The listing builds one solid part. Answer for the finished solid, in the listing's coordinates (mm). A direction names the side the tool comes from. Give positions to 0.01 mm unless a question says otherwise; leave off trailing zeros. Loops run counter-clockwise (first coordinate to the right, second up) from the corner with the lowest first, then second, coordinate; pieces in that order, holes last.
Item 1: Section B-B, the plane z = 19.05 is taken. Give the vertices of the cut face in (x, y), and give its area (3 significant figures).
Item 2: A tool of negligible diameter and unlimited length cuts with its end or side. For faces 1 (the face through (10.878, 1, 9)), 2 (the face through (-6.6, 2, 0)), 3 (the face through (17, 2.2, 21)), from which of +Z, -Z, +X, -X, +Y, -Y can it reach the whole face along a straight path? Write none if from no direction.
Item 3: Section C-C, the plane x = 0 is taken. Give the vertices of the cut face in (y, z).
Item 4: Consider line 1 along Z through (x, y) = (19.05, 1.3); line 2 along X through (y, z) = (3.25, -17.5). Determine where each line is inside the solid, lowest interval first.
Item 5: Section D-D, the plane z = 8.5 is taken. Give the vertices of the cut face in (x, y).
Item 6: The mould has two halves that part along Z. Classify faces 4 (the face through (-24.19, 2.54, -24.15)), 5 (the face through (10.878, 1, -9)): pulls with the +Z half, pulls with the -Z half, needs draft (parallel to the pull), parting line crosses it, or undercut.
Item 7: Each of these flat-tipped pins is pushed along its axis until it touches: pin 1 Ø6 at (x, z) = (19.05, 19.05) entering from +Y; pin 2 Ø1.6 at (x, z) = (8, -7) entering from -Y. Where does it stop, or does it pass through?
Item 8: Section A-A, the plane x = 19.05 is taken. Give the vertices of the cut face in (y, z), and give its area (3 significant figures).
from build123d import *

# Parameters (mm, degrees)
SKETCH1_W           = 50.1
SKETCH1_H           = 50.1
SKETCH1_R           = 1.7
SKETCH1_R_2         = 2.5527
SKETCH1_W_2         = 13.2
SKETCH1_H_2         = 6.8
BOSS_EXTRUDE1_DEPTH = 5
FILLET1_R           = 3
CUT_EXTRUDE1_DEPTH  = 2.6
SKETCH5_R           = 4.5675
CUT_EXTRUDE4_DEPTH  = 2.8
FILLET2_R           = 0.5


with BuildPart() as part:
    # Sketch1 → Boss-Extrude1 (new body)
    with BuildSketch(Plane(origin=(0, 0, 0), x_dir=(1, 0, 0), z_dir=(0, 1, 0))):
        Rectangle(SKETCH1_W, SKETCH1_H)
        with Locations(Location((8.128, 8.5344, 0), (0, 0, 270))):
            Circle(SKETCH1_R, mode=Mode.SUBTRACT)
        with Locations(Location((-8.128, 8.5344, 0), (0, 0, 270))):
            Circle(SKETCH1_R, mode=Mode.SUBTRACT)
        with Locations(Location((19.05, 19.05, 0), (0, 0, 270))):
            Circle(SKETCH1_R_2, mode=Mode.SUBTRACT)
        with Locations(Location((-19.05, 19.05, 0), (0, 0, 270))):
            Circle(SKETCH1_R_2, mode=Mode.SUBTRACT)
        with Locations(Location((19.05, -19.05, 0), (0, 0, 270))):
            Circle(SKETCH1_R_2, mode=Mode.SUBTRACT)
        with Locations(Location((-19.05, -19.05, 0), (0, 0, 270))):
            Circle(SKETCH1_R_2, mode=Mode.SUBTRACT)
        with Locations(Location((8.128, -8.5344, 0), (0, 0, 270))):
            Circle(SKETCH1_R, mode=Mode.SUBTRACT)
        with Locations(Location((-8.128, -8.5344, 0), (0, 0, 270))):
            Circle(SKETCH1_R, mode=Mode.SUBTRACT)
        Rectangle(SKETCH1_W_2, SKETCH1_H_2, mode=Mode.SUBTRACT)
    extrude(amount=BOSS_EXTRUDE1_DEPTH)

    # Fillet1
    fillet1_edges = [part.edges().sort_by_distance(p)[0] for p in [
        (-25.05, 2.5, 25.05),
        (-25.05, 2.5, -25.05),
        (25.05, 2.5, -25.05),
        (25.05, 2.5, 25.05),
    ]]
    fillet(fillet1_edges, radius=FILLET1_R)

    # Sketch2 → Cut-Extrude1 (cut)
    with BuildSketch(Plane.XZ):
        Polygon((-8.128, 11.709826481), (-10.878, 10.12211324), (-10.878, 6.94668676), (-8.128, 5.358973519), (-5.378, 6.94668676), (-5.378, 10.12211324), align=None)
        Polygon((8.128, 11.709826481), (5.378, 10.12211324), (5.378, 6.94668676), (8.128, 5.358973519), (10.878, 6.94668676), (10.878, 10.12211324), align=None)
        Polygon((-8.128, -5.358973519), (-10.878, -6.94668676), (-10.878, -10.12211324), (-8.128, -11.709826481), (-5.378, -10.12211324), (-5.378, -6.94668676), align=None)
        Polygon((8.128, -5.358973519), (5.378, -6.94668676), (5.378, -10.12211324), (8.128, -11.709826481), (10.878, -10.12211324), (10.878, -6.94668676), align=None)
    extrude(amount=-CUT_EXTRUDE1_DEPTH, mode=Mode.SUBTRACT)

    # Sketch5 → Cut-Extrude4 (cut)
    with BuildSketch(Plane(origin=(0, 5, 0), x_dir=(1, 0, 0), z_dir=(0, 1, 0))):
        with Locations(Location((-19.05, 19.05, 0), (0, 0, 270))):
            Circle(SKETCH5_R)
        with Locations(Location((19.05, 19.05, 0), (0, 0, 270))):
            Circle(SKETCH5_R)
        with Locations(Location((19.05, -19.05, 0), (0, 0, 270))):
            Circle(SKETCH5_R)
        with Locations(Location((-19.05, -19.05, 0), (0, 0, 270))):
            Circle(SKETCH5_R)
    extrude(amount=-CUT_EXTRUDE4_DEPTH, mode=Mode.SUBTRACT)

    # Fillet2
    fillet2_edges = [part.edges().sort_by_distance(p)[0] for p in [
        (-19.05, 5, 14.4825),
        (19.05, 5, 14.4825),
        (19.05, 5, -23.6175),
        (-19.05, 5, -23.6175),
    ]]
    fillet(fillet2_edges, radius=FILLET2_R)


solid = part.part
Worked answers:
1. outline: (-25.05, 0) - (-21.6, 0) - (-21.6, 2.2) - (-23.62, 2.2) - (-23.62, 4.5) arc R0.5 ccw to (-24.12, 5) - (-25.05, 5) - close; (-16.5, 0) - (16.5, 0) - (16.5, 2.2) - (14.48, 2.2) - (14.48, 4.5) arc R0.5 ccw to (13.98, 5) - (-13.98, 5) arc R0.5 ccw to (-14.48, 4.5) - (-14.48, 2.2) - (-16.5, 2.2) - close; (21.6, 0) - (25.05, 0) - (25.05, 5) - (24.12, 5) arc R0.5 ccw to (23.62, 4.5) - (23.62, 2.2) - (21.6, 2.2) - close
1. area: 177 mm2
2. face 1: -Y
2. face 2: +Y, -Y
2. face 3: +Y
3. outline: (0, -25.05) - (5, -25.05) - (5, -3.4) - (0, -3.4) - close; (0, 3.4) - (5, 3.4) - (5, 25.05) - (0, 25.05) - close
4. line 1: z = -25.05 to -21.6, -16.5 to 16.5, 21.6 to 25.05
4. line 2: x = -25.05 to -23.35, -14.75 to 14.75, 23.35 to 25.05
5. outline: (-25.05, 0) - (-10.88, 0) - (-10.88, 2.6) - (-9.83, 2.6) - (-9.83, 5) - (-25.05, 5) - close; (-6.43, 2.6) - (-5.38, 2.6) - (-5.38, 0) - (5.38, 0) - (5.38, 2.6) - (6.43, 2.6) - (6.43, 5) - (-6.43, 5) - close; (9.83, 2.6) - (10.88, 2.6) - (10.88, 0) - (25.05, 0) - (25.05, 5) - (9.83, 5) - close
6. face 4: pulls with the -Z half
6. face 5: undercut
7. pin 1: stops at y = 2.2
7. pin 2: stops at y = 2.6
8. outline: (0, -25.05) - (5, -25.05) - (5, -24.12) arc R0.5 ccw to (4.5, -23.62) - (2.2, -23.62) - (2.2, -21.6) - (0, -21.6) - close; (0, -16.5) - (2.2, -16.5) - (2.2, -14.48) - (4.5, -14.48) arc R0.5 ccw to (5, -13.98) - (5, 13.98) arc R0.5 ccw to (4.5, 14.48) - (2.2, 14.48) - (2.2, 16.5) - (0, 16.5) - close; (0, 21.6) - (2.2, 21.6) - (2.2, 23.62) - (4.5, 23.62) arc R0.5 ccw to (5, 24.12) - (5, 25.05) - (0, 25.05) - close
8. area: 177 mm2
